Input: dimensioned drawing with shaded views. Units: mm. Origin: part minimum x, y, z. A direction names the side the tool comes from. Give positions to 0.01 mm unless a question says otherwise; leave off trailing zeros. Loops run counter-clockwise (first coordinate to the right, second up) from the corner with the lowest first, then second, coordinate; pieces in that order, holes last. Notation, with made-up numbers: M 80.25,65 L 131.25,65 A15 ccw 131.25,69 Z; hole C 21.5,-31.5 d9. An arc over 180 degrees is marked long. Use CSV: the item, a comma, the result in double quotes. Start each with the question number.
Q1. Section B-B, the plane x = 10. Output: boundary loops of the cut face in (y, z), plus the area to 3 significant figures.
Q2. Section A-A, the plane z = 25. Output: boundary loops of the cut face in (x, y).
Q3. Section C-C, the plane y = 8. Output: boundary loops of the cut face in (x, z), plus the area to 3 significant figures.
Q4. Reachability of the marked faces 1, 2 and 3 from +Z, -Z, +X, -X, +Y, -Y: full face, straight path, thin tool, end or side. Return the list, or none.
Q5. Section D-D, the plane x = 4.5. Output: boundary loops of the cut face in (y, z), plus the area to 3 significant figures.
Q6. Pin query (flat end, axial travel): pin 1 (4 mm diameter, centred on y = 13, z = 14.5, fed in from +X); pin 2 (6 mm diameter, centred on x = 3.5, y = 6.5, fed in from -Z); pin 3 (2 mm diameter, centred on x = 2.5, y = 6.5, fed in from +Z); pin 4 (1.2 mm diameter, centred on x = 2, z = 12.5, fed in from -Y). Return the tip coordinate at first contact, or that it passes through.
Q7. Material intervals for line 1 along Z through (x, y) = (6.75, 8.25); line 2 along Y through (x, z) = (9.5, 25); line 3 along X through (y, z) = (14.25, 8.25), sorted ascending.
Q8. Pull-direction query (Y, two-part tool) for the marked faces 4, 5 and 6; classes: released by +Y, released by -Y, zero draft, split by the parting line, or undercut.
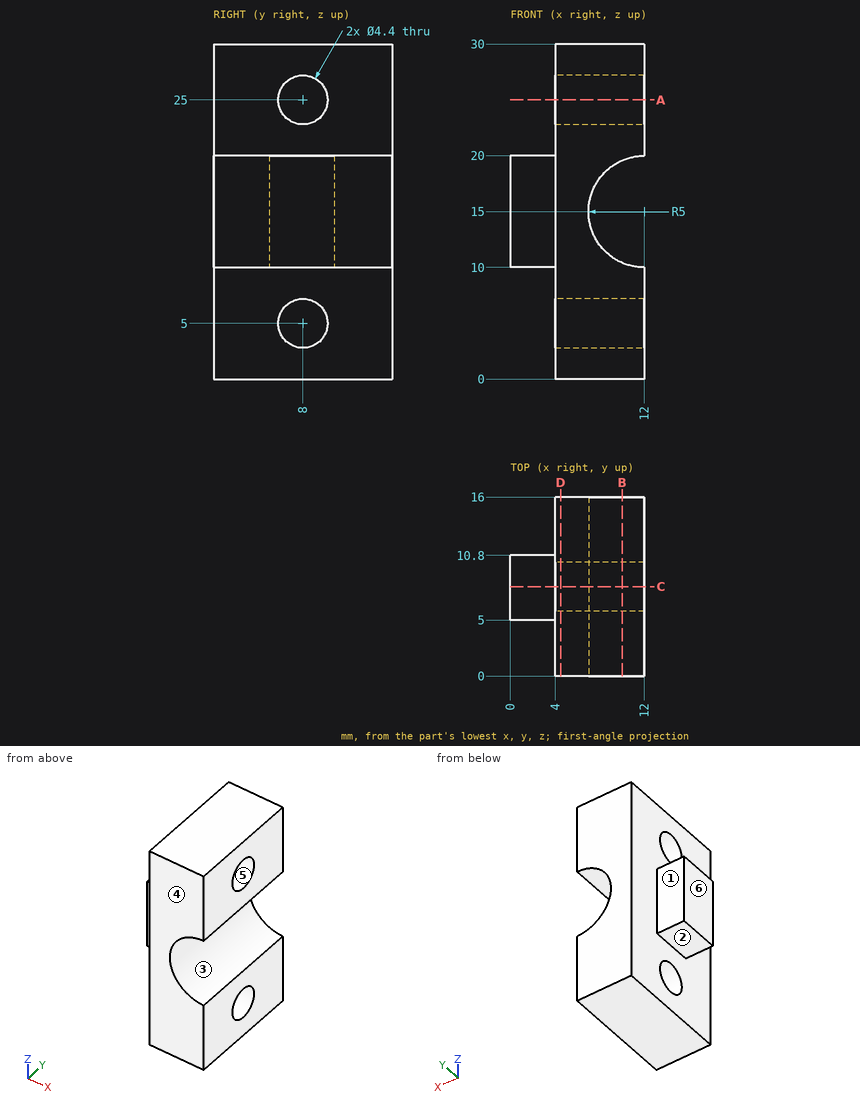
A:
1,outline,"M 0,0 L 16,0 L 16,10.42 L 0,10.42 Z; M 0,19.58 L 16,19.58 L 16,30 L 0,30 Z; hole C 8,5 d4.4; hole C 8,25 d4.4"
1,area,"303 mm^2"
2,outline,"M 4,0 L 12,0 L 12,5.8 L 4,5.8 Z; M 4,10.2 L 12,10.2 L 12,16 L 4,16 Z"
3,outline,"M 0,10 L 4,10 L 4,7.2 L 12,7.2 L 12,10 A5 cw 12,20 L 12,22.8 L 4,22.8 L 4,20 L 0,20 Z; M 4,0 L 12,0 L 12,2.8 L 4,2.8 Z; M 4,27.2 L 12,27.2 L 12,30 L 4,30 Z"
3,area,"170 mm^2"
4,face 1,"+Z, -Z, -X, +Y"
4,face 2,"-Z, -X, +Y, -Y"
4,face 3,"+X, +Y, -Y"
5,outline,"M 0,0 L 16,0 L 16,30 L 0,30 Z; hole C 8,5 d4.4; hole C 8,25 d4.4"
5,area,"450 mm^2"
6,pin 1,"x = 7.67"
6,pin 2,"z = 0"
6,pin 3,"z = 20"
6,pin 4,"y = 5"
7,line 1,"0 to 2.81, 7.19 to 22.81, 27.19 to 30"
7,line 2,"0 to 5.8, 10.2 to 16"
7,line 3,"4 to 12"
8,face 4,"released by -Y"
8,face 5,"undercut"
8,face 6,"zero draft"
